```python
from build123d import *

# Parameters (mm, degrees)
SKETCH1_R           = 40
BOSS_EXTRUDE2_DEPTH = 110
SKETCH4_R           = 15
BOSS_EXTRUDE3_DEPTH = 50
SKETCH5_R           = 15
BOSS_EXTRUDE4_DEPTH = 50
SKETCH6_R           = 30
CUT_EXTRUDE1_DEPTH  = 100
SKETCH8_W           = 31
SKETCH8_H           = 5
CUT_EXTRUDE2_DEPTH  = 100


with BuildPart() as part:
    # Sketch1 → Boss-Extrude2 (new body)
    with BuildSketch(Plane.XY):
        Circle(SKETCH1_R)
    extrude(amount=BOSS_EXTRUDE2_DEPTH)

    # Sketch3 → Revolve1 (revolve)
    with BuildSketch(Plane(origin=(0, 0, 0), x_dir=(0, 0, -1), z_dir=(1, 0, 0))):
        with BuildLine():
            Line((0, 40), (0, -40))
            ThreePointArc((0, -40), (40, 0), (0, 40))
        make_face()
    revolve(axis=Axis((0, -40, 0), (0, 1, 0)))

    # Sketch4 → Boss-Extrude3 (add)
    with BuildSketch(Plane(origin=(0, 0, 0), x_dir=(1, 0, 0), z_dir=(0, 1, 0))):
        Circle(SKETCH4_R)
    extrude(amount=BOSS_EXTRUDE3_DEPTH)

    # Sketch5 → Boss-Extrude4 (add)
    with BuildSketch(Plane(origin=(0, 0, 0), x_dir=(1, 0, 0), z_dir=(0, 1, 0))):
        Circle(SKETCH5_R)
    extrude(amount=-BOSS_EXTRUDE4_DEPTH)

    # Sketch6 → Cut-Extrude1 (cut)
    with BuildSketch(Plane.XY.offset(110)):
        Circle(SKETCH6_R)
    extrude(amount=-CUT_EXTRUDE1_DEPTH, mode=Mode.SUBTRACT)

    # Sketch8 → Cut-Extrude2 (cut)
    with BuildSketch(Plane.XY.offset(110)):
        with Locations((15.5, 0)):
            Rectangle(SKETCH8_W, SKETCH8_H)
    extrude(amount=-CUT_EXTRUDE2_DEPTH, mode=Mode.SUBTRACT)


solid = part.part
```
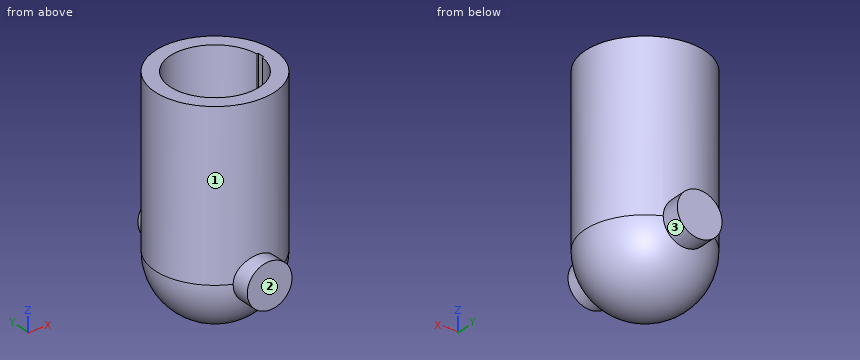
Geometry check sheet. Reference: the model listing, model coordinates, mm. Face numbers are marked on the shaded views. A direction names the side the tool comes from. Give positions to 0.01 mm unless a question says otherwise; leave off trailing zeros. Loops run counter-clockwise (first coordinate to the right, second up) from the corner with the lowest first, then second, coordinate; pieces in that order, holes last. Notation, with made-up numbers: M -39.5,84.5 L -11.5,84.5 A19 cw -11.5,100.5 Z; hole C 9,-39 d5. An arc over 180 degrees is marked long. Answer as CSV lines item,"result".
Item 1: Cross-section at D-D on y = -43. Record the cut outline in (x, z).
Values:
outline,"C 0,0 d30"
Item 2: Cross-section at B-B on y = 13. Record the cut outline in (x, z).
Values:
outline,"M -37.83,0 A37.83 ccw 37.83,0 L 37.83,110 L 27.04,110 L 27.04,10 L -27.04,10 L -27.04,110 L -37.83,110 Z"
Item 3: Cross-section at C-C on x = 0. Record the cut outline in (y, z).
Values:
outline,"M -50,-15 L -37.08,-15 A40 ccw 37.08,-15 L 50,-15 L 50,15 L 40,15 L 40,110 L 30,110 L 30,10 L -30,10 L -30,110 L -40,110 L -40,15 L -50,15 Z"
Item 4: Material ranges on line 1 (Y direction, x = 0, z = 46.5); line 2 (X direction, y = -19.5, z = 98.5); line 3 (X direction, y = 24.5, z = 34), recorded low to high.
Values:
line 1,"y = -40 to -30, 30 to 40"
line 2,"x = -34.92 to -22.8, 22.8 to 34.92"
line 3,"x = -31.62 to -17.31, 17.31 to 31.62"
Item 5: Depth check by flat-ended pin: P1, Ø0.9, axis at x = 30.5, z = 47, coming from the +Y side; P2, Ø6, axis at x = -23, y = 26, coming from the -Z side; P3, Ø4, axis at x = -4, y = 28, coming from the -Z side. Enter the tip coordinate at first touch or a pass-through.
Values:
P1,"stops at y = 26.4"
P2,"stops at z = -24.38"
P3,"stops at z = -30.15"
Item 6: Cross-section at A-A on z = 86. Record the cut outline in (x, y), and give its area (3 significant figures).
Values:
outline,"C 0,0 d80; hole M 29.9,-2.5 L 31,-2.5 L 31,2.5 L 29.9,2.5 A30 ccw long Z"
area,"2,190 mm²"
Item 7: Access from +Z, -Z, +X, -X, +Y, -Y to the whole of each face (thin tool, end or side, straight path). Record for the marked faces 1, 2 and 3.
Values:
face 1,"+Z"
face 2,"+Z, -Z, +X, -X, -Y"
face 3,"+Y"
